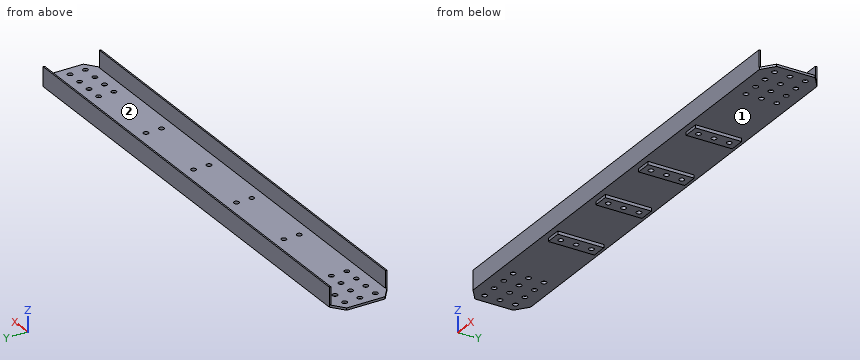
```python
from build123d import *

# Parameters (mm, degrees)
SKETCH_1_R          = 13
EXTRUDE_725_DEPTH   = 11.5
SKETCH_2_W          = 2408.049034164
SKETCH_2_H          = 7.5
EXTRUDE_1_DEPTH     = 89
SKETCH_3_W          = 80
SKETCH_3_H          = 240
EXTRUDE_2_DEPTH     = 16
SKETCH_4_R          = 13
CUT_EXTRUDE_1_DEPTH = 1308.983562588


with BuildPart() as part:
    # 草图1 → Extrude 725 (new body)
    with BuildSketch(Plane.XY):
        Polygon((-1205, 0), (1205, 0), (1270, 50), (1270, 250), (1205, 300), (-1205, 300), (-1270, 250), (-1270, 50), align=None)
        with Locations((-1220, 230)):
            Circle(SKETCH_1_R, mode=Mode.SUBTRACT)
        with Locations((-1220, 150)):
            Circle(SKETCH_1_R, mode=Mode.SUBTRACT)
        with Locations((-1140, 230)):
            Circle(SKETCH_1_R, mode=Mode.SUBTRACT)
        with Locations((-1140, 150)):
            Circle(SKETCH_1_R, mode=Mode.SUBTRACT)
        with Locations((-1060, 230)):
            Circle(SKETCH_1_R, mode=Mode.SUBTRACT)
        with Locations((-1060, 150)):
            Circle(SKETCH_1_R, mode=Mode.SUBTRACT)
        with Locations((-980, 150)):
            Circle(SKETCH_1_R, mode=Mode.SUBTRACT)
        with Locations(Location((-1060, 70, 0), (0, 0, 180))):
            Circle(SKETCH_1_R, mode=Mode.SUBTRACT)
        with Locations(Location((-1140, 70, 0), (0, 0, 180))):
            Circle(SKETCH_1_R, mode=Mode.SUBTRACT)
        with Locations(Location((-1220, 70, 0), (0, 0, 180))):
            Circle(SKETCH_1_R, mode=Mode.SUBTRACT)
        with Locations((1220, 70)):
            Circle(SKETCH_1_R, mode=Mode.SUBTRACT)
        with Locations((1140, 70)):
            Circle(SKETCH_1_R, mode=Mode.SUBTRACT)
        with Locations((1060, 70)):
            Circle(SKETCH_1_R, mode=Mode.SUBTRACT)
        with Locations(Location((980, 150, 0), (0, 0, 180))):
            Circle(SKETCH_1_R, mode=Mode.SUBTRACT)
        with Locations(Location((1060, 150, 0), (0, 0, 180))):
            Circle(SKETCH_1_R, mode=Mode.SUBTRACT)
        with Locations(Location((1060, 230, 0), (0, 0, 180))):
            Circle(SKETCH_1_R, mode=Mode.SUBTRACT)
        with Locations(Location((1140, 150, 0), (0, 0, 180))):
            Circle(SKETCH_1_R, mode=Mode.SUBTRACT)
        with Locations(Location((1140, 230, 0), (0, 0, 180))):
            Circle(SKETCH_1_R, mode=Mode.SUBTRACT)
        with Locations(Location((1220, 150, 0), (0, 0, 180))):
            Circle(SKETCH_1_R, mode=Mode.SUBTRACT)
        with Locations(Location((1220, 230, 0), (0, 0, 180))):
            Circle(SKETCH_1_R, mode=Mode.SUBTRACT)
        with Locations((-980, 70)):
            Circle(SKETCH_1_R, mode=Mode.SUBTRACT)
        with Locations((-980, 230)):
            Circle(SKETCH_1_R, mode=Mode.SUBTRACT)
        with Locations((980, 70)):
            Circle(SKETCH_1_R, mode=Mode.SUBTRACT)
        with Locations((980, 230)):
            Circle(SKETCH_1_R, mode=Mode.SUBTRACT)
    extrude(amount=-EXTRUDE_725_DEPTH)

    # 草图2 → 凸台-拉伸1 (add)
    with BuildSketch(Plane.XY):
        with Locations((-0.975482918, 296.25)):
            Rectangle(SKETCH_2_W, SKETCH_2_H)
        with Locations((-0.975482918, 3.75)):
            Rectangle(SKETCH_2_W, SKETCH_2_H)
    extrude(amount=EXTRUDE_1_DEPTH)

    # 草图3 → 凸台-拉伸2 (add)
    with BuildSketch(Plane(origin=(0, 0, -11.5), x_dir=(-1, 0, 0), z_dir=(0, 0, -1))):
        with Locations((-580, 150)):
            Rectangle(SKETCH_3_W, SKETCH_3_H)
        with Locations((-180, 150)):
            Rectangle(SKETCH_3_W, SKETCH_3_H)
        with Locations((180, 150)):
            Rectangle(SKETCH_3_W, SKETCH_3_H)
        with Locations((580, 150)):
            Rectangle(SKETCH_3_W, SKETCH_3_H)
    extrude(amount=EXTRUDE_2_DEPTH)

    # 草图4 → 切除-拉伸1 (cut, through all)
    with BuildSketch(Plane.XY):
        with Locations((-580, 230)):
            Circle(SKETCH_4_R)
        with Locations((-580, 150)):
            Circle(SKETCH_4_R)
        with Locations((-180, 230)):
            Circle(SKETCH_4_R)
        with Locations((-180, 150)):
            Circle(SKETCH_4_R)
        with Locations(Location((-180, 70, 0), (0, 0, 180))):
            Circle(SKETCH_4_R)
        with Locations(Location((-580, 70, 0), (0, 0, 180))):
            Circle(SKETCH_4_R)
        with Locations((580, 70)):
            Circle(SKETCH_4_R)
        with Locations((180, 70)):
            Circle(SKETCH_4_R)
        with Locations(Location((180, 150, 0), (0, 0, 180))):
            Circle(SKETCH_4_R)
        with Locations(Location((180, 230, 0), (0, 0, 180))):
            Circle(SKETCH_4_R)
        with Locations(Location((580, 150, 0), (0, 0, 180))):
            Circle(SKETCH_4_R)
        with Locations(Location((580, 230, 0), (0, 0, 180))):
            Circle(SKETCH_4_R)
    extrude(amount=-CUT_EXTRUDE_1_DEPTH, mode=Mode.SUBTRACT)


solid = part.part
```
Source: CAD feature listing. Evaluate the final solid. Frame: model axes, mm. Face numbers are marked on the shaded views. Coordinates: 2 decimals unless noted, no trailing zeros. Write each loop counter-clockwise with the first axis right and the second up, starting at its lowest first coordinate (ties: lowest second). Pieces come first, ordered by that corner, then holes. Notation, with made-up numbers: (-27.75, -6.5) -> (-17.75, -6.5) arc R11 cw to (-17.75, 10.5) -> close; hole circle Ø7 at (68, -1). An arc over 180 degrees is marked (long way). Return JSON: item names as keys, results as strings. Group by question number.
1) Section query B-B, the plane y = 189. Return loops of the section in (x, z).
2) Mould query, pull axis Y, two halves, no side actions, for the marked faces 1 and 2. Classes: +Y half, -Y half, draft (parallel to the pull), parting line (faces both ways), or undercut.
3) Section query A-A, the plane z = 31.5. Return loops of the section in (x, y), plus the area to 3 significant figures.
4) Contact query for flat-ended pins moving along their axis: P1, Ø8, axis at x = -913, z = -16, coming from the +Y side; P2, Ø2, axis at y = 4, z = 34, coming from the +X side; P3, Ø2, axis at x = -294, y = 116, coming from the -Z side; P4, Ø13, axis at x = 180, z = -20.5, coming from the -Y side. Output: stop coordinate, or through.
5) Ray query, line 1 along X through (y, z) = (101.5, -13); line 2 along Y through (x, z) = (-980, -7); line 3 along Y through (x, z) = (-588, 50.5). Return the intervals inside material, ascending.
6) Section query C-C, the plane x = -321. Return loops of the section in (y, z), plus the area to 4 significant figures.
From the geometry:
{
 "1": {"outline": "(-1270, -11.5) -> (-620, -11.5) -> (-620, -27.5) -> (-540, -27.5) -> (-540, -11.5) -> (-220, -11.5) -> (-220, -27.5) -> (-140, -27.5) -> (-140, -11.5) -> (140, -11.5) -> (140, -27.5) -> (220, -27.5) -> (220, -11.5) -> (540, -11.5) -> (540, -27.5) -> (620, -27.5) -> (620, -11.5) -> (1270, -11.5) -> (1270, 0) -> (-1270, 0) -> close"},
 "2": {"face 1": "draft", "face 2": "undercut"},
 "3": {"outline": "(-1205, 0) -> (1203.05, 0) -> (1203.05, 7.5) -> (-1205, 7.5) -> close; (-1205, 292.5) -> (1203.05, 292.5) -> (1203.05, 300) -> (-1205, 300) -> close", "area": "36,100 mm²"},
 "4": {"P1": "through", "P2": "x = 1203.05", "P3": "z = -11.5", "P4": "y = 30"},
 "5": {"line 1": "-620 to -540, -220 to -140, 140 to 220, 540 to 620", "line 2": "0 to 57, 83 to 137, 163 to 217, 243 to 300", "line 3": "0 to 7.5, 292.5 to 300"},
 "6": {"outline": "(0, -11.5) -> (300, -11.5) -> (300, 89) -> (292.5, 89) -> (292.5, 0) -> (7.5, 0) -> (7.5, 89) -> (0, 89) -> close", "area": "4,785 mm²"}
}
